Check sheet for the modelled part. Datum: model origin and axes. Units: mm. A direction names the side the tool comes from. Round coordinates to 2 decimals unless told otherwise and drop trailing zeros. Write each loop counter-clockwise with the first axis right and the second up, starting at its lowest first coordinate (ties: lowest second). Pieces come first, ordered by that corner, then holes. Notation, with made-up numbers: (88.25, 47) -> (146.25, 47) arc R30 ccw to (146.25, 77) -> close; hole circle Ø8 at (36.25, 48). An arc over 180 degrees is marked (long way). Write item = value, one per line.
from build123d import *

# Parameters (mm, degrees)
SKETCH1_R             = 6
BOSS_EXTRUDE1_DEPTH   = 174
CHAMFER1_SIZE         = 1
M5_TAPPED_HOLE1_D     = 4.2
M5_TAPPED_HOLE1_DEPTH = 14
M5_TAPPED_HOLE1_TIP   = 1.2618073
CHAMFER2_SIZE         = 0.5
M5_TAPPED_HOLE2_D     = 4.2
M5_TAPPED_HOLE2_DEPTH = 14
M5_TAPPED_HOLE2_TIP   = 1.2618073
CHAMFER3_SIZE         = 0.5


with BuildPart() as part:
    # Sketch1 → Boss-Extrude1 (new body)
    with BuildSketch(Plane(origin=(0, 0, 0), x_dir=(0, 0, -1), z_dir=(1, 0, 0))):
        Circle(SKETCH1_R)
    extrude(amount=BOSS_EXTRUDE1_DEPTH)

    # Chamfer1
    chamfer1_edges = [part.edges().sort_by_distance(p)[0] for p in [
        (0, 0, 6),
        (174, 0, 6),
    ]]
    chamfer(chamfer1_edges, length=CHAMFER1_SIZE)

    # M5 Tapped Hole1
    with Locations(Plane(origin=(174, 0, 0), x_dir=(0, 0, -1), z_dir=(1, 0, 0))):
        with Locations((0, 0)):
            Hole(M5_TAPPED_HOLE1_D / 2, depth=M5_TAPPED_HOLE1_DEPTH)
            with Locations((0, 0, -(M5_TAPPED_HOLE1_DEPTH + M5_TAPPED_HOLE1_TIP / 2))):  # 118° drill point
                Cone(0, M5_TAPPED_HOLE1_D / 2, M5_TAPPED_HOLE1_TIP, mode=Mode.SUBTRACT)

    # Chamfer2
    chamfer2_edges = [part.edges().sort_by_distance(p)[0] for p in [
        (174, 0, -2.1),
    ]]
    chamfer(chamfer2_edges, length=CHAMFER2_SIZE)

    # M5 Tapped Hole2
    with Locations(Plane.ZY):
        with Locations((0, 0)):
            Hole(M5_TAPPED_HOLE2_D / 2, depth=M5_TAPPED_HOLE2_DEPTH)
            with Locations((0, 0, -(M5_TAPPED_HOLE2_DEPTH + M5_TAPPED_HOLE2_TIP / 2))):  # 118° drill point
                Cone(0, M5_TAPPED_HOLE2_D / 2, M5_TAPPED_HOLE2_TIP, mode=Mode.SUBTRACT)

    # Chamfer3
    chamfer3_edges = [part.edges().sort_by_distance(p)[0] for p in [
        (0, 0, 2.1),
    ]]
    chamfer(chamfer3_edges, length=CHAMFER3_SIZE)


solid = part.part
(1) Go/stop test with flat-tipped pins: P1, Ø4, axis at x = 104, y = -4.5, coming from the +Z side; P2, Ø1, axis at x = 102.5, y = -2.5, coming from the +Z side; P3, Ø2.5, axis at y = 0, z = 0, coming from the -X side. Record where each tip stops, or that it passes through.
Worked answers:
P1 = 5.45
P2 = 5.66
P3 = 14.51
(2) Sectioned sample at A-A on x = 72. Enter the section's corners in (y, z).
Worked answers:
outline = circle Ø12 at (0, 0)
(3) Material ranges on L1, parallel to Y at x = 7, z = 0; L2, parallel to Z at x = 98, y = -0.75; L3, parallel to X at y = -2, z = 5.25, recorded low to high. Write a range as [from, to].
Worked answers:
L1 = [-6, -2.1], [2.1, 6]
L2 = [-5.95, 5.95]
L3 = [0.62, 173.38]
(4) Release check for a two-part mould opening along Y. For faces 4 (the flat face through (174, -2, -2)), 5 (the cylindrical face through (86, 0, 6)), 6 (the conical face through (158.96, -0.14, -0.34)) record: pulls with the +Y half, pulls with the -Y half, needs draft (parallel to the pull), parting line crosses it, or undercut.
Worked answers:
face_4 = needs draft
face_5 = parting line crosses it
face_6 = undercut
(5) Access from +Z, -Z, +X, -X, +Y, -Y to the whole of each face (thin tool, end or side, straight path). Record for faces 1 (the flat face through (0, -2, -2)), 2 (the cylindrical face through (166.656, 0.631, 2.003)), 3 (the cylindrical face through (7.344, 0.631, -2.003)).
Worked answers:
face_1 = +Z, -Z, -X, +Y, -Y
face_2 = +X
face_3 = -X
